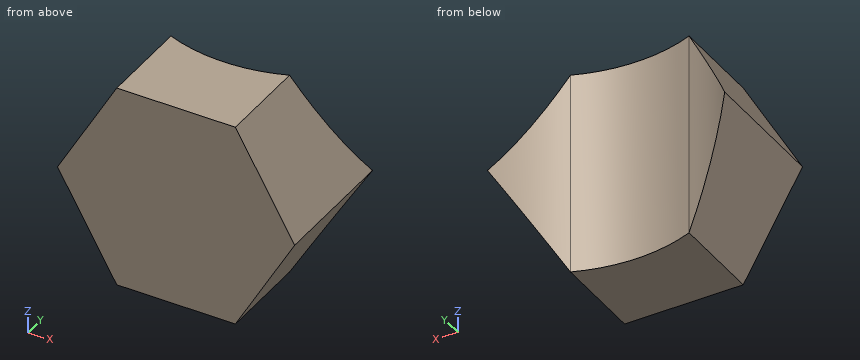
```python
from build123d import *

# Parameters (mm, degrees)
F1_DEPTH = 9
F3_DEPTH = 25


with BuildPart() as f1:
    # F0 (on Front) → F1 (new body)
    with BuildSketch(Plane.XZ):
        Polygon((2.193931, 3.8), (-2.193931, 3.8), (-4.387862, 0), (-2.193931, -3.8), (2.193931, -3.8), (4.387862, 0), align=None)
    extrude(amount=F1_DEPTH)

    # F2 (on face) → F3 (cut)
    with BuildSketch(Plane.XY.offset(3.8)):
        with BuildLine():
            Line((-2.193931, 0), (-2.193931, -5.584502))
            ThreePointArc((-2.193931, -5.584502), (0, -6), (2.193931, -5.584502))
            Line((2.193931, -5.584502), (2.193931, 0))
            Line((2.193931, 0), (-2.193931, 0))
        make_face()
        with BuildLine():
            ThreePointArc((2.193931, -5.584502), (4.958003, -3.379084), (6, 0))
            ThreePointArc((6, 0), (-3.379084, 4.958003), (-2.193931, -5.584502))
            Line((-2.193931, -5.584502), (-2.193931, 0))
            Line((-2.193931, 0), (2.193931, 0))
            Line((2.193931, 0), (2.193931, -5.584502))
        make_face()
    extrude(amount=-F3_DEPTH, mode=Mode.SUBTRACT)


solid = f1.part
```
Source: CAD feature listing. Evaluate the final solid. Frame: model axes, mm. Round coordinates to 2 decimals unless told otherwise and drop trailing zeros. Write each loop counter-clockwise with the first axis right and the second up, starting at its lowest first coordinate (ties: lowest second). Pieces come first, ordered by that corner, then holes. Notation, with made-up numbers: M 20.25,55 L 33.25,55 A27 cw 33.25,85 Z; hole C -18.5,-8 d7. An arc over 180 degrees is marked long. Answer as a JSON object with one key per item and string values. Group by question number.
(1) Ray query, line 1 (Z direction, x = 2.25, y = -7.35); line 2 (X direction, y = -6.2, z = -2); line 3 (Y direction, x = 0.75, z = 2.25). Return the intervals inside material, ascending. Write a range as [from, to].
(2) Section query B-B on y = -4.85. Output: boundary loops of the cut face in (x, z).
(3) Section query A-A on y = -6.65. Output: boundary loops of the cut face in (x, z), then the cut area to 3 significant figures.
(4) First-contact query: pin 1 (1.5 mm diameter, centred on y = -5, z = 3, fed in from -X); pin 2 (1 mm diameter, centred on y = -5.5, z = 1.5, fed in from +X). Flat tips, straight axial feed; report the tip coordinate or a pass-through.
(5) Section query D-D on x = 0. Output: boundary loops of the cut face in (y, z), then the cut area to 3 significant figures.
(6) Section query C-C on z = 1.25. Output: boundary loops of the cut face in (x, y), then the cut area to 3 significant figures.
Computed values:
{
 "1": {"line 1": "[-3.7, 3.7]", "line 2": "[-3.23, 3.23]", "line 3": "[-9, -5.95]"},
 "2": {"outline": "M -4.39,0 L -3.53,-1.48 L -3.53,1.48 Z; M 3.53,-1.48 L 4.39,0 L 3.53,1.48 Z"},
 "3": {"outline": "M -4.39,0 L -2.19,-3.8 L 2.19,-3.8 L 4.39,0 L 2.19,3.8 L -2.19,3.8 Z", "area": "50.0 mm^2"},
 "4": {"pin 1": "x = -3.08", "pin 2": "x = 3.81"},
 "5": {"outline": "M -9,-3.8 L -6,-3.8 L -6,3.8 L -9,3.8 Z", "area": "22.8 mm^2"},
 "6": {"outline": "M -3.67,-9 L 3.67,-9 L 3.67,-4.75 A6 cw 2.19,-5.58 A6 cw -2.19,-5.58 A6 cw -3.67,-4.75 Z", "area": "24.9 mm^2"}
}
